from build123d import *

# Parameters (mm, degrees)
BOSS_EXTRUDE1_DEPTH = 3.175
SKETCH2_R           = 2.5
CUT_EXTRUDE1_DEPTH  = 4.175


with BuildPart() as part:
    # Sketch1 → Boss-Extrude1 (new body)
    with BuildSketch(Plane.XY):
        with BuildLine():
            Line((-125.176151208, 25.103095989), (-36.276151208, 25.103095989))
            ThreePointArc((-36.276151208, 25.103095989), (-31.786023147, 23.24322405), (-29.926151208, 18.753095989))
            Line((-29.926151208, 18.753095989), (-29.926151208, -120.946904011))
            ThreePointArc((-29.926151208, -120.946904011), (-31.786023147, -125.437032071), (-36.276151208, -127.296904011))
            Line((-36.276151208, -127.296904011), (-125.176151208, -127.296904011))
            ThreePointArc((-125.176151208, -127.296904011), (-129.666279268, -125.437032071), (-131.526151208, -120.946904011))
            Line((-131.526151208, -120.946904011), (-131.526151208, 18.753095989))
            ThreePointArc((-131.526151208, 18.753095989), (-129.666279268, 23.24322405), (-125.176151208, 25.103095989))
        make_face()
        with BuildLine():
            Line((-131.526151208, -49.826904011), (-131.526151208, -26.966904011))
            Line((-131.526151208, -26.966904011), (-175.976151208, -26.966904011))
            ThreePointArc((-175.976151208, -26.966904011), (-180.466279268, -28.82677595), (-182.326151208, -33.316904011))
            Line((-182.326151208, -33.316904011), (-182.326151208, -43.476904011))
            ThreePointArc((-182.326151208, -43.476904011), (-180.466279268, -47.967032071), (-175.976151208, -49.826904011))
            Line((-175.976151208, -49.826904011), (-131.526151208, -49.826904011))
        make_face()
        with BuildLine():
            Line((14.523848792, -26.966904011), (-29.926151208, -26.966904011))
            Line((-29.926151208, -26.966904011), (-29.926151208, -75.226904011))
            Line((-29.926151208, -75.226904011), (14.523848792, -75.226904011))
            ThreePointArc((14.523848792, -75.226904011), (19.013976853, -73.367032071), (20.873848792, -68.876904011))
            Line((20.873848792, -68.876904011), (20.873848792, -33.316904011))
            ThreePointArc((20.873848792, -33.316904011), (19.013976853, -28.82677595), (14.523848792, -26.966904011))
        make_face()
    extrude(amount=BOSS_EXTRUDE1_DEPTH)

    # Sketch2 → Cut-Extrude1 (cut, through all)
    with BuildSketch(Plane.XY.offset(3.175)):
        with Locations((-169.626151208, -38.396904011)):
            Circle(SKETCH2_R)
        with Locations((8.173848792, -63.796904011)):
            Circle(SKETCH2_R)
        with Locations((-156.926151208, -38.396904011)):
            Circle(SKETCH2_R)
        with Locations((-144.226151208, -38.396904011)):
            Circle(SKETCH2_R)
        with Locations((-4.526151208, -63.796904011)):
            Circle(SKETCH2_R)
        with Locations((-17.226151208, -63.796904011)):
            Circle(SKETCH2_R)
        with Locations((-4.526151208, -51.096904011)):
            Circle(SKETCH2_R)
        with Locations((-17.226151208, -51.096904011)):
            Circle(SKETCH2_R)
        with Locations((-4.526151208, -38.396904011)):
            Circle(SKETCH2_R)
        with Locations((-17.226151208, -38.396904011)):
            Circle(SKETCH2_R)
        with Locations((8.173848792, -51.096904011)):
            Circle(SKETCH2_R)
        with Locations((8.173848792, -38.396904011)):
            Circle(SKETCH2_R)
    extrude(amount=-CUT_EXTRUDE1_DEPTH, mode=Mode.SUBTRACT)


solid = part.part
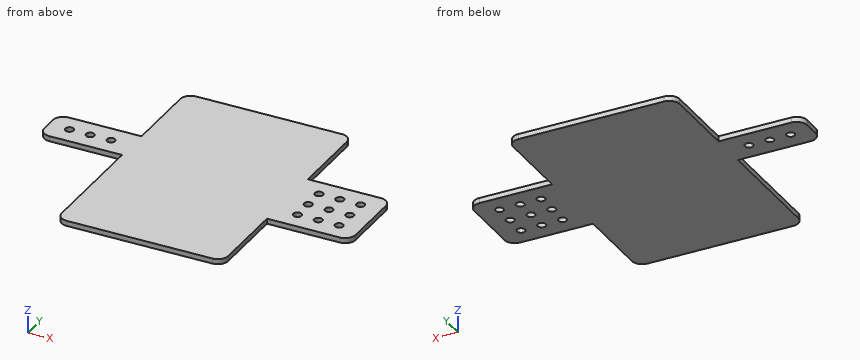
CAD build for the part. Positions are in the model's coordinates, mm. Coordinates: 2 decimals unless noted, no trailing zeros. Order: outer loops, then holes, each group sorted by start corner. A loop starts at its lowest first (then second) coordinate and runs counter-clockwise, first axis right, second up. Notation, with made-up numbers: (4, 2.5) -> (49, 2.5) arc R20 cw to (49, 9.5) -> close; hole circle Ø6 at (-29.75, 81.25). An arc over 180 degrees is marked (long way). Answer in a Markdown table with one row per item.
1) Band-saw the part on A-A (x = 8.5). List the corners of the cut face in (y, z) (3 decimals).
Check values:
| item | result |
|---|---|
| outline | (-75.227, 0) -> (-66.276, 0) -> (-66.276, 3.175) -> (-75.227, 3.175) -> close; (-61.318, 0) -> (-53.576, 0) -> (-53.576, 3.175) -> (-61.318, 3.175) -> close; (-48.618, 0) -> (-40.876, 0) -> (-40.876, 3.175) -> (-48.618, 3.175) -> close; (-35.918, 0) -> (-26.967, 0) -> (-26.967, 3.175) -> (-35.918, 3.175) -> close |
2) Band-saw the part on C-C (y = -18). List the corners of the cut face in (x, z) (3 decimals), and give its area (3 significant figures).
Check values:
| item | result |
|---|---|
| outline | (-131.526, 0) -> (-29.926, 0) -> (-29.926, 3.175) -> (-131.526, 3.175) -> close |
| area | 323 mm2 |
3) Flat gauge pins, fed straight in: P1, Ø1, axis at x = -140, z = 1.5, coming from the +Y side; P2, Ø3, axis at x = -17.23, y = -51.1, coming from the +Z side; P3, Ø1, axis at y = -88.5, z = 2, coming from the +X side. Where does each tip first touch, or does it go through?
Check values:
| item | result |
|---|---|
| P1 | y = -26.97 |
| P2 | through |
| P3 | x = -29.93 |
4) Drill centre lines: line 1 (X direction, y = -109, z = 1.7); line 2 (X direction, y = -66.5, z = 1.1); line 3 (Y direction, x = 4, z = 2.9). Where is each one in solid material? Low to high.
Check values:
| item | result |
|---|---|
| line 1 | -131.53 to -29.93 |
| line 2 | -131.53 to 20.87 |
| line 3 | -75.23 to -26.97 |
5) Band-saw the part on B-B (z = 2.6). Give the number of separate pieces and of enclosed holes in the cut face, and give its area (3 significant figures).
Check values:
| item | result |
|---|---|
| separate pieces | 1 |
| enclosed holes | 12 |
| area | 18,800 mm2 |
